Here's how the part is built. I have some questions about the finished solid (model axes, mm). A direction names the side the tool comes from. Give positions to 0.01 mm unless a question says otherwise; leave off trailing zeros. Write each loop counter-clockwise with the first axis right and the second up, starting at its lowest first coordinate (ties: lowest second). Pieces come first, ordered by that corner, then holes. Notation, with made-up numbers: (-3.5, 23.25) -> (0.5, 23.25) arc R20 ccw to (0.5, 47.25) -> close; hole circle Ø6 at (86.25, 82.5). An arc over 180 degrees is marked (long way). Return JSON: item names as keys, results as strings.
from build123d import *
from OCP.BRepFilletAPI import BRepFilletAPI_MakeChamfer

# Parameters (mm, degrees)
ESQUISSE1_W                                       = 9
ESQUISSE1_H                                       = 6.5
BOSS_EXTRU_1_DEPTH                                = 150
ENL_V_MAT_EXTRU_1_DEPTH                           = 301.051349772
CHANFREIN1_SIZE                                   = 0.3
CONG_1_R                                          = 0.2
CHANFREIN2_SIZE                                   = 0.1
CHANFREIN2_SIZE2                                  = 0.167315719
CHAMBRAGE_POUR_VIS_SIX_PANS_CREUX_M31_D           = 3.6
CHAMBRAGE_POUR_VIS_SIX_PANS_CREUX_M31_CBORE_D     = 6.5
CHAMBRAGE_POUR_VIS_SIX_PANS_CREUX_M31_CBORE_DEPTH = 3.8
R_P_TITION_LIN_AIRE1_COUNT                        = 15
R_P_TITION_LIN_AIRE1_PITCH                        = 20


with BuildPart() as part:
    # Esquisse1 → Boss.-Extru.1 (new, symmetric)
    with BuildSketch(Plane.XY):
        Rectangle(ESQUISSE1_W, ESQUISSE1_H)
    extrude(amount=BOSS_EXTRU_1_DEPTH, both=True)

    # Esquisse2 → Enlèv. mat.-Extru.1 (cut, through all)
    with BuildSketch(Plane(origin=(0, 0, -150), x_dir=(-1, 0, 0), z_dir=(0, 0, -1))):
        Polygon((-4.5, 1.968382141), (-3.9, 1.75), (-3.9, 1.15), (-4.5, 0.931617859), align=None)
    enl_v_mat_extru_1 = extrude(amount=-ENL_V_MAT_EXTRU_1_DEPTH, mode=Mode.SUBTRACT)

    # Symétrie1: Enlèv. mat.-Extru.1 across plane
    add(enl_v_mat_extru_1.mirror(Plane(origin=(0, 0, 0), x_dir=(0, 0, 1), z_dir=(1, 0, 0))), mode=Mode.SUBTRACT)

    # Chanfrein1
    chanfrein1_edges = [part.edges().sort_by_distance(p)[0] for p in [
        (-4.5, 3.25, 0),
        (4.5, 3.25, 0),
        (4.5, -3.25, 0),
        (-4.5, -3.25, 0),
    ]]
    chamfer(chanfrein1_edges, length=CHANFREIN1_SIZE)

    # Congé1
    cong_1_edges = [part.edges().sort_by_distance(p)[0] for p in [
        (3.9, 1.75, 0),
        (3.9, 1.15, 0),
        (-3.9, 1.15, 0),
        (-3.9, 1.75, 0),
    ]]
    fillet(cong_1_edges, radius=CONG_1_R)

    # Chanfrein2: one chamfer whose edges measure the first distance from different faces: ONE call of the kernel's chamfer builder (chamfer() names one face for all edges)
    chanfrein2_edges_1 = [part.edges().sort_by_distance(p)[0] for p in [
        (4.5, 0.931617859, 0),
    ]]
    chanfrein2_side_1 = [part.faces().sort_by_distance(p)[0] for p in [
        (4.5, -1.00919107, 0),
    ]]
    chanfrein2_edges_2 = [part.edges().sort_by_distance(p)[0] for p in [
        (4.5, 1.968382141, 0),
    ]]
    chanfrein2_side_2 = [part.faces().sort_by_distance(p)[0] for p in [
        (4.265797986, 1.883139579, 0),
    ]]
    chanfrein2_edges_3 = [part.edges().sort_by_distance(p)[0] for p in [
        (-4.5, 1.968382141, 0),
    ]]
    chanfrein2_side_3 = [part.faces().sort_by_distance(p)[0] for p in [
        (-4.5, 2.45919107, 0),
    ]]
    chanfrein2_edges_4 = [part.edges().sort_by_distance(p)[0] for p in [
        (-4.5, 0.931617859, 0),
    ]]
    chanfrein2_side_4 = [part.faces().sort_by_distance(p)[0] for p in [
        (-4.265797986, 1.016860421, 0),
    ]]
    chanfrein2 = BRepFilletAPI_MakeChamfer(part.part.solid().wrapped)
    for e in chanfrein2_edges_1:
        chanfrein2.Add(CHANFREIN2_SIZE, CHANFREIN2_SIZE2, e.wrapped, chanfrein2_side_1[0].wrapped)  # the first distance lies on this face
    for e in chanfrein2_edges_2:
        chanfrein2.Add(CHANFREIN2_SIZE, CHANFREIN2_SIZE2, e.wrapped, chanfrein2_side_2[0].wrapped)  # the first distance lies on this face
    for e in chanfrein2_edges_3:
        chanfrein2.Add(CHANFREIN2_SIZE, CHANFREIN2_SIZE2, e.wrapped, chanfrein2_side_3[0].wrapped)  # the first distance lies on this face
    for e in chanfrein2_edges_4:
        chanfrein2.Add(CHANFREIN2_SIZE, CHANFREIN2_SIZE2, e.wrapped, chanfrein2_side_4[0].wrapped)  # the first distance lies on this face
    add(Compound.cast(chanfrein2.Shape()), mode=Mode.REPLACE)

    # Chambrage pour vis à six pans creux M31 (through all)
    with Locations(Plane(origin=(0, 3.25, 0), x_dir=(1, 0, 0), z_dir=(0, 1, 0))):
        with Locations((0, 140)):
            chambrage_pour_vis_six_pans_creux_m31 = CounterBoreHole(CHAMBRAGE_POUR_VIS_SIX_PANS_CREUX_M31_D / 2, CHAMBRAGE_POUR_VIS_SIX_PANS_CREUX_M31_CBORE_D / 2, CHAMBRAGE_POUR_VIS_SIX_PANS_CREUX_M31_CBORE_DEPTH)

    # Répétition linéaire1: Chambrage pour vis à six pans creux M31 ×15
    with Locations(*[(0, 0, i * R_P_TITION_LIN_AIRE1_PITCH) for i in range(1, R_P_TITION_LIN_AIRE1_COUNT)]):
        add(chambrage_pour_vis_six_pans_creux_m31, mode=Mode.SUBTRACT)


solid = part.part
1. Suppose I cut it at A-A, the plane y = -1.75. Count the separate pieces of the cut face and the enclosed holes in it, and give its area (3 significant figures).
Taken from the geometry:
{"separate pieces": "1", "enclosed holes": "15", "area": "2,550 mm²"}
2. If we mould it in two halves opening along X, with no side actions, what happens to faces 3 (the face through (3, 3.25, 2)), 4 (the face through (-0.705, 1.377, 83.173)), 5 (the face through (1.4, -0.55, -38.6))? For each: released by +X, released by -X, zero draft, split by the parting line, or undercut.
Taken from the geometry:
{"face 3": "zero draft", "face 4": "undercut", "face 5": "undercut"}
3. Suppose I cut it at B-B, the plane z = -91.5. List the corners of the cut face in (x, y) for me.
Taken from the geometry:
{"outline": "(-4.5, -2.95) -> (-4.2, -3.25) -> (4.2, -3.25) -> (4.5, -2.95) -> (4.5, 0.83) -> (4.34, 0.99) -> (4.03, 1.1) arc R0.2 cw to (3.9, 1.29) -> (3.9, 1.61) arc R0.2 cw to (4.03, 1.8) -> (4.41, 1.93) -> (4.5, 2.14) -> (4.5, 2.95) -> (4.2, 3.25) -> (-4.2, 3.25) -> (-4.5, 2.95) -> (-4.5, 2.07) -> (-4.34, 1.91) -> (-4.03, 1.8) arc R0.2 cw to (-3.9, 1.61) -> (-3.9, 1.29) arc R0.2 cw to (-4.03, 1.1) -> (-4.41, 0.97) -> (-4.5, 0.76) -> close"}
4. For pin 1 Ø2 at (x, z) = (1, -60.5) entering from +Y, with a flat end and sliding along its axis, tell me the tip position at first contact or that it passes through.
Taken from the geometry:
{"pin 1": "stops at y = -0.55"}
5. If I drill on line 1 (X direction, y = -2.35, z = 140); line 2 (Y direction, x = -4, z = 16); line 3 (X direction, y = 1.25, z = -74.5), over which ranges is the centre line in solid material (lowest first)? Write a range as [from, to].
Taken from the geometry:
{"line 1": "x = [-4.5, -1.8], [1.8, 4.5]", "line 2": "y = [-3.25, 1.12], [1.78, 3.25]", "line 3": "x = [-3.9, 3.9]"}
6. Which directions (+Z, -Z, +X, -X, +Y, -Y) give clear straight access to the entire face, cutting with the end or side of a thin tool? Please do faces 1 (the face through (-2.579, 1.377, 1.978)), 2 (the face through (0, -3.25, 2)).
Taken from the geometry:
{"face 1": "+Y", "face 2": "+Z, -Z, +X, -X, -Y"}
